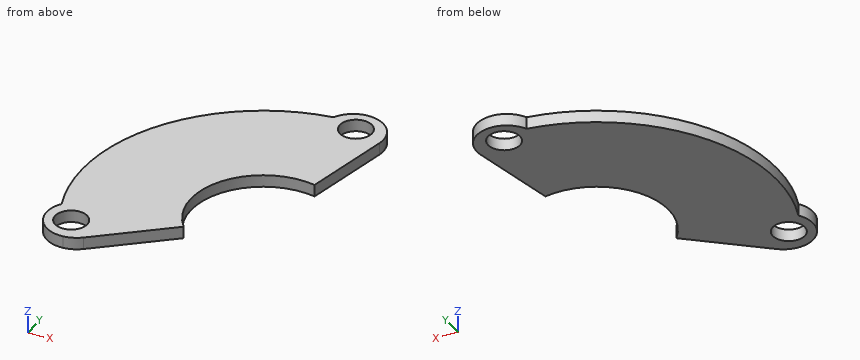
from build123d import *

# Parameters (mm, degrees)
SKETCH_1_R          = 7.18
EXTRUDE_1_DEPTH     = 1.2
SKETCH_2_R          = 1.6
CUT_EXTRUDE_1_DEPTH = 10
CUT_EXTRUDE_START   = -11.2
CUT_EXTRUDE_4_DEPTH = 11.2


with BuildPart() as part:
    # 草图1 → 凸台-拉伸1 (new body)
    with BuildSketch(Plane.XY):
        with BuildLine():
            ThreePointArc((-14.058374697, -11.241089844), (0, -18), (14.058374697, -11.241089844))
            ThreePointArc((14.058374697, -11.241089844), (16.887495374, -9.75), (16.76425672, -6.554364701))
            ThreePointArc((16.76425672, -6.554364701), (15.588457268, 9), (2.705882023, 17.795454545))
            ThreePointArc((2.705882023, 17.795454545), (0, 19.5), (-2.705882023, 17.795454545))
            ThreePointArc((-2.705882023, 17.795454545), (-15.588457268, 9), (-16.76425672, -6.554364701))
            ThreePointArc((-16.76425672, -6.554364701), (-16.887495374, -9.75), (-14.058374697, -11.241089844))
        make_face()
        Circle(SKETCH_1_R, mode=Mode.SUBTRACT)
    extrude(amount=EXTRUDE_1_DEPTH)

    # 草图2 → 切除-拉伸1 (cut)
    with BuildSketch(Plane.XY.offset(1.2)):
        with Locations((0, 17)):
            Circle(SKETCH_2_R)
        with Locations((14.722431864, -8.5)):
            Circle(SKETCH_2_R)
        with Locations((-14.722431864, -8.5)):
            Circle(SKETCH_2_R)
    extrude(amount=-CUT_EXTRUDE_1_DEPTH, mode=Mode.SUBTRACT)

    # 草图4 → 切除-拉伸4 (cut)
    with BuildSketch(Plane.XY.offset(11.2).offset(CUT_EXTRUDE_START)):
        with BuildLine():
            Line((0, 0), (2.949996498, 15.954545455))
            ThreePointArc((2.949996498, 15.954545455), (0.928512003, 19.352694421), (-2.705882023, 17.795454545))
            Line((-2.705882023, 17.795454545), (-0.609984312, 23.633101635))
            Line((-0.609984312, 23.633101635), (9.450831052, 25.36709559))
            Line((9.450831052, 25.36709559), (30.272136365, -16.841499514))
            Line((30.272136365, -16.841499514), (-5.709784057, -19.189026381))
            Line((-5.709784057, -19.189026381), (-25.420914817, -11.863123573))
            Line((-25.420914817, -11.863123573), (-16.76425672, -6.554364701))
            ThreePointArc((-16.76425672, -6.554364701), (-16.295668999, -10.480462193), (-12.34204342, -10.532044636))
            Line((-12.34204342, -10.532044636), (0, 0))
        make_face()
    extrude(amount=CUT_EXTRUDE_4_DEPTH, mode=Mode.SUBTRACT)


solid = part.part
Check sheet for the modelled part. Datum: model origin and axes. Units: mm. Give positions to 0.01 mm unless a question says otherwise; leave off trailing zeros. Loops run counter-clockwise (first coordinate to the right, second up) from the corner with the lowest first, then second, coordinate; pieces in that order, holes last. Notation, with made-up numbers: M 44,12 L 83,12 A13 cw 83,37 Z; hole C 43.5,71 d1. An arc over 180 degrees is marked long. Return JSON: item names as keys, results as strings. Group by question number.
1. Cross-section at D-D on x = -10.75. Record the boundary of the cut face in (y, z), plus the area to 3 significant figures.
2. Go/stop test with a flat-tipped pin: pin 1 (1.9 mm diameter, centred on x = -14.72, y = -8.5, fed in from +Z). Record where the tip stops, or that it passes through.
3. Thickness scan on L1, parallel to Y at x = 0, z = 0.5; L2, parallel to Y at x = -16, z = 0.2; L3, parallel to Y at x = -9.5, z = 0.9. Record the ranges inside material, lowest first.
4. Cross-section at A-A on x = -14.5. Record the boundary of the cut face in (y, z), plus the area to 3 significant figures.
5. Cross-section at B-B on z = 0.25. Record the boundary of the cut face in (x, y), plus the area to 3 significant figures.
6. Cross-section at C-C on y = -8.5. Record the boundary of the cut face in (x, z).
Return value:
{
 "1": {"outline": "M -9.17,0 L 14.44,0 L 14.44,1.2 L -9.17,1.2 Z", "area": "28.3 mm^2"},
 "2": {"pin 1": "through"},
 "3": {"L1": "7.18 to 15.4, 18.6 to 19.5", "L2": "-10.71 to -9.46, -7.54 to 8.25", "L3": "-8.11 to 15.29"},
 "4": {"outline": "M -11.24,0 L -10.08,0 L -10.08,1.2 L -11.24,1.2 Z; M -6.92,0 L 10.67,0 L 10.67,1.2 L -6.92,1.2 Z", "area": "22.5 mm^2"},
 "5": {"outline": "M -16.76,-6.55 A3 ccw -12.34,-10.53 L -5.46,-4.66 A7.18 cw 1.31,7.06 L 2.95,15.95 A3 ccw -2.71,17.8 A18 ccw Z; hole C -14.72,-8.5 d3.2; hole C 0,17 d3.2", "area": "330 mm^2"},
 "6": {"outline": "M -17.28,0 L -16.32,0 L -16.32,1.2 L -17.28,1.2 Z; M -13.12,0 L -9.96,0 L -9.96,1.2 L -13.12,1.2 Z"}
}
